Input: dimensioned drawing with shaded views. Units: mm. Origin: part minimum x, y, z. Give positions to 0.01 mm unless a question says otherwise; leave off trailing zeros. Loops run counter-clockwise (first coordinate to the right, second up) from the corner with the lowest first, then second, coordinate; pieces in that order, holes last.
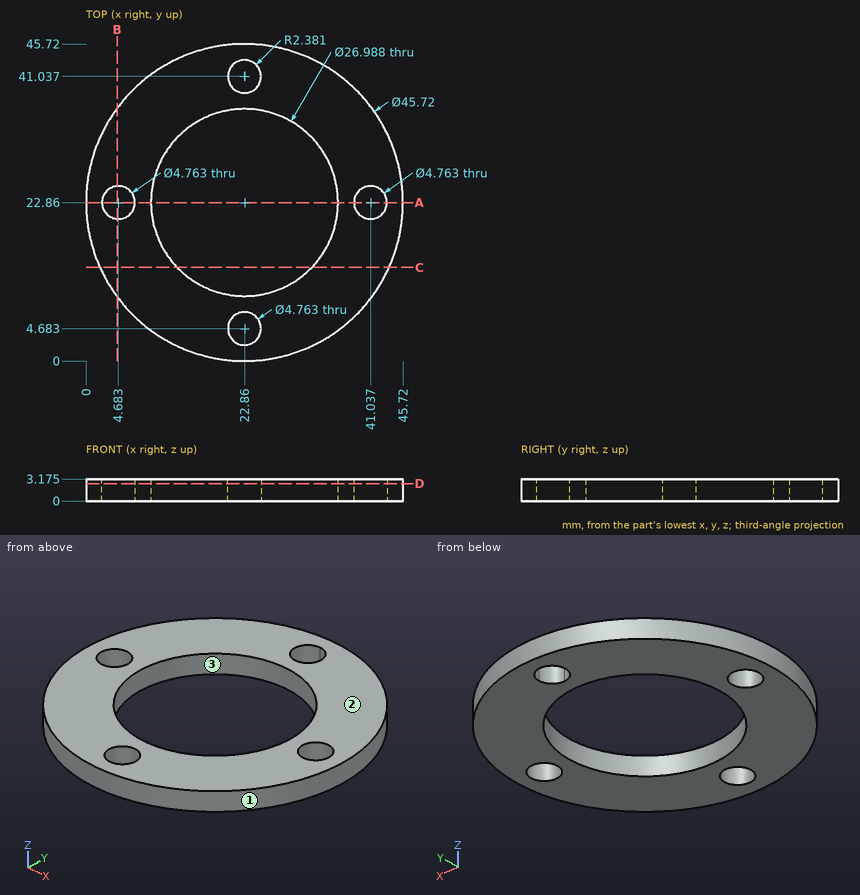
(1) Mould query, pull axis X, two halves, no side actions, for the marked faces 1, 2 and 3. Classes: pulls with the +X half, pulls with the -X half, needs draft (parallel to the pull), parting line crosses it, or undercut.
A:
face 1: parting line crosses it
face 2: needs draft
face 3: undercut
(2) Section C-C, the plane y = 13.5. Return the cut outline in (x, z) (1 decimal).
A:
outline: (2, 0) - (13.1, 0) - (13.1, 3.2) - (2, 3.2) - close; (32.6, 0) - (43.7, 0) - (43.7, 3.2) - (32.6, 3.2) - close
(3) Section A-A, the plane y = 22.86. Return the cut outline in (x, z) (1 decimal).
A:
outline: (0, 0) - (2.3, 0) - (2.3, 3.2) - (0, 3.2) - close; (7.1, 0) - (9.4, 0) - (9.4, 3.2) - (7.1, 3.2) - close; (36.4, 0) - (38.7, 0) - (38.7, 3.2) - (36.4, 3.2) - close; (43.4, 0) - (45.7, 0) - (45.7, 3.2) - (43.4, 3.2) - close
(4) Section B-B, the plane x = 4.5. Return the cut outline in (y, z) (1 decimal).
A:
outline: (9.2, 0) - (20.5, 0) - (20.5, 3.2) - (9.2, 3.2) - close; (25.2, 0) - (36.5, 0) - (36.5, 3.2) - (25.2, 3.2) - close
(5) Section D-D, the plane z = 2.5. Return the cut outline in (x, y) (1 decimal).
A:
outline: circle Ø45.7 at (22.9, 22.9); hole circle Ø4.8 at (4.7, 22.9); hole circle Ø27 at (22.9, 22.9); hole circle Ø4.8 at (22.9, 4.7); hole circle Ø4.8 at (22.9, 41); hole circle Ø4.8 at (41, 22.9)
(6) Ray query, line 1 along Y through (x, z) = (22.86, 1.4) (1 decimal); line 2 along Y through (x, z) = (24, 2.5) (1 decimal); line 3 along X through (y, z) = (32, 1) (1 decimal). Return the intervals inside material, ascending.
A:
line 1: y = 0 to 2.3, 7.1 to 9.4, 36.4 to 38.7, 43.4 to 45.7
line 2: y = 0 to 2.6, 6.8 to 9.4, 36.3 to 38.9, 43.1 to 45.7
line 3: x = 1.9 to 12.9, 32.8 to 43.8
